from build123d import *

# Parameters (mm, degrees)
SKETCH1_W           = 40
SKETCH1_H           = 40
BOSS_EXTRUDE1_DEPTH = 2
SKETCH2_W           = 30
SKETCH2_H           = 30
SKETCH2_W_2         = 26
SKETCH2_H_2         = 26
BOSS_EXTRUDE2_DEPTH = 3
FILLET1_R           = 0.5


with BuildPart() as part:
    # Sketch1 → Boss-Extrude1 (new body)
    with BuildSketch(Plane.XY):
        with Locations((-5.192307692, -4.855769231)):
            Rectangle(SKETCH1_W, SKETCH1_H)
    extrude(amount=BOSS_EXTRUDE1_DEPTH)

    # Sketch2 → Boss-Extrude2 (add)
    with BuildSketch(Plane.XY.offset(2)):
        with Locations((-5.192307692, -4.855769231)):
            Rectangle(SKETCH2_W, SKETCH2_H)
        with Locations((-5.192307692, -4.855769231)):
            Rectangle(SKETCH2_W_2, SKETCH2_H_2, mode=Mode.SUBTRACT)
    extrude(amount=BOSS_EXTRUDE2_DEPTH)

    # Fillet1
    fillet1_edges = [part.edges().sort_by_distance(p)[0] for p in [
        (-20.192307692, -4.855769231, 5),
        (-5.192307692, -19.855769231, 5),
        (9.807692308, -4.855769231, 5),
        (-5.192307692, 10.144230769, 5),
        (-18.192307692, -4.855769231, 5),
        (-5.192307692, -17.855769231, 5),
        (7.807692308, -4.855769231, 5),
        (-5.192307692, 8.144230769, 5),
    ]]
    fillet(fillet1_edges, radius=FILLET1_R)


solid = part.part
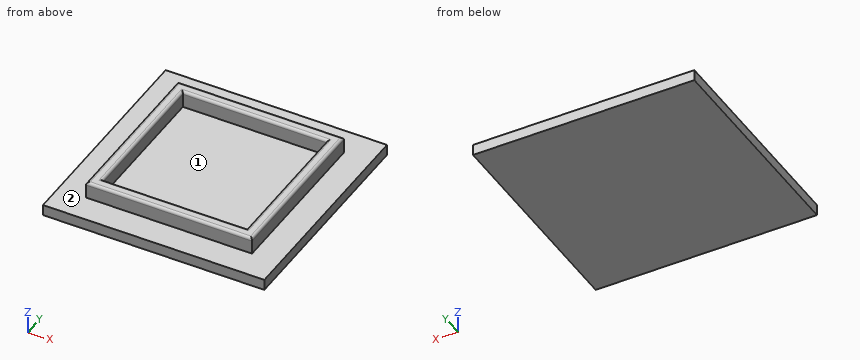
Design review of the part built by this model. Coordinates are the model's own, in mm. Face numbers are marked on the shaded views. Give positions to 0.01 mm unless a question says otherwise; leave off trailing zeros. Loops run counter-clockwise (first coordinate to the right, second up) from the corner with the lowest first, then second, coordinate; pieces in that order, holes last. Notation, with made-up numbers: M 50,-19.75 L 72,-19.75 A22 ccw 72,-13.75 Z; hole C -10.5,-34 d11. An arc over 180 degrees is marked long. Write item = value, one per line.
Q1. We need section C-C (x = -8). Give the boundary of the cut face in (y, z).
Output values:
outline = M -24.86,0 L 15.14,0 L 15.14,2 L 10.14,2 L 10.14,4.5 A0.5 ccw 9.64,5 L 8.64,5 A0.5 ccw 8.14,4.5 L 8.14,2 L -17.86,2 L -17.86,4.5 A0.5 ccw -18.36,5 L -19.36,5 A0.5 ccw -19.86,4.5 L -19.86,2 L -24.86,2 Z
Q2. We need section B-B (y = -7.5). Give the boundary of the cut face in (x, z).
Output values:
outline = M -25.19,0 L 14.81,0 L 14.81,2 L 9.81,2 L 9.81,4.5 A0.5 ccw 9.31,5 L 8.31,5 A0.5 ccw 7.81,4.5 L 7.81,2 L -18.19,2 L -18.19,4.5 A0.5 ccw -18.69,5 L -19.69,5 A0.5 ccw -20.19,4.5 L -20.19,2 L -25.19,2 Z
Q3. We need section A-A (z = 3.45). Give the boundary of the cut face in (x, y).
Output values:
outline = M -20.19,-19.86 L 9.81,-19.86 L 9.81,10.14 L -20.19,10.14 Z; hole M -18.19,-17.86 L 7.81,-17.86 L 7.81,8.14 L -18.19,8.14 Z
Q4. Insertion check: pin 1 (2 mm diameter, centred on y = -8.5, z = 3.5, fed in from +X); pin 2 (1.5 mm diameter, centred on y = -17.5, z = 3, fed in from -X); pin 3 (2 mm diameter, centred on x = 1, z = 3.5, fed in from -Y). Each pin has a flat end and moves straight along its axis. Give the tip position at first contact, or say it passes through.
Output values:
pin_1 = 9.81
pin_2 = -20.19
pin_3 = -19.86
Q5. To check wall thickness, follow line 1 (Y direction, x = 0, z = 3.8); line 2 (X direction, y = -8, z = 4.35); line 3 (X direction, y = -19.5, z = 2.25). State the ranges of each line that lie inside material, in increasing order. Write a range as [from, to].
Output values:
line_1 = [-19.86, -17.86], [8.14, 10.14]
line_2 = [-20.19, -18.19], [7.81, 9.81]
line_3 = [-20.19, 9.81]
Q6. Draft analysis for pull direction Y (two halves, no side actions). For the marked faces 1 and 2, state which applies: +Y half, -Y half, draft (parallel to the pull), parting line (faces both ways), or undercut.
Output values:
face_1 = undercut
face_2 = draft
Q7. We need section D-D (x = 11). Give the boundary of the cut face in (y, z), plus the area to 3 significant figures.
Output values:
outline = M -24.86,0 L 15.14,0 L 15.14,2 L -24.86,2 Z
area = 80.0 mm^2
